The listing builds one solid part. Answer for the finished solid, in the listing's coordinates (mm). A direction names the side the tool comes from. Coordinates: 2 decimals unless noted, no trailing zeros. Order: outer loops, then holes, each group sorted by start corner. A loop starts at its lowest first (then second) coordinate and runs counter-clockwise, first axis right, second up. Notation, with made-up numbers: (65.25, -38) - (88.25, -38) arc R25 ccw to (88.25, -2) - close; hole circle Ø3 at (34.5, 67). An arc over 180 degrees is marked (long way). Use one line per item in the form item = value. Start each with the question number.
Item 1: Section B-B, the plane y = 9.75 is taken. Write down the section's boundary in (x, z).
Item 2: A tool of negligible diameter and unlimited length cuts with its end or side. For faces 1 (the flat face through (0, 10, -2)), 2 (the flat face through (0, -3, 0)), from which of +Z, -Z, +X, -X, +Y, -Y can it reach the whole face along a straight path? Write none if from no direction.
Item 3: Each of these flat-tipped pins is pushed along its axis until it touches: pin 1 Ø1.5 at (y, z) = (2, -1) entering from -X; pin 2 Ø3.5 at (x, y) = (0, 11) entering from -Z; pin 3 Ø1.1 at (x, z) = (1, -2.5) entering from +Y; pin 4 Ø3 at (y, z) = (7.5, 2) entering from +X. Where does it stop, or does it pass through?
Item 4: Consider line 1 along Y through (x, z) = (-1.5, -2.5); line 2 along Z through (x, y) = (2, 8.75); line 3 along X through (y, z) = (9, 2). Determine where each line is inside the solid, lowest interval first. Write a range as [from, to].
Item 5: Section A-A, the plane y = 2.25 is taken. Write down the section's boundary in (x, z).
Autodesk Inventor part; units mm, degrees
ref_plane "YZ Plane" through (0, 0, 0) normal (1, 0, 0) x (0, 1, 0)
ref_plane "XZ Plane" through (0, 0, 0) normal (0, 1, 0) x (-1, 0, 0)
ref_plane "XY Plane" through (0, 0, 0) normal (0, 0, 1) x (1, 0, 0)
sketch "スケッチ1" plane through (0, 0, 0) normal (0, 1, 0) x (-1, 0, 0)
  circle A0 centre (0, 0) radius 3
  dimension "d0" = 6
extrude "押し出し1" add sketch "スケッチ1" along normal blind 4
sketch "スケッチ2" plane through (0, 4, 0) normal (0, 1, 0) x (1, 0, 0)
  circle A0 centre (0, 0) radius 3
  line L0 (0, 3) -> (0, 2)
  line L1 (0, 2) -> (2.2361, 2)
  arc A1 (-2.2361, 2) -> (2.2361, 2) centre (0, 0) ccw
  line L2 (-2.2361, 2) -> (0, 2)
  dimension "d3" = 1
extrude "押し出し2" add sketch "スケッチ2" along normal blind 12 contours A0 L2 L1
sketch "スケッチ3" plane through (0, 0, 0) normal (0, -1, 0) x (1, 0, 0)
  circle A0 centre (0, 0) radius 3
extrude "押し出し3" add sketch "スケッチ3" along normal blind 3
fillet "フィレット1" radius 0.4 1 edges at (0, 16, 3)
properties part number "モーター100：1軸"
Response:
q1.outline = (-2.24, -2) - (2.24, -2) arc R3 ccw (long way) to start
q2.face_1 = -Z, +X, -X, +Y
q2.face_2 = +Z, -Z, +X, -X, -Y
q3.pin_1 = -2.99
q3.pin_2 = -2
q3.pin_3 = 16
q3.pin_4 = 2.96
q4.line_1 = [-3, 4]
q4.line_2 = [-2, 2.24]
q4.line_3 = [-2.24, 2.24]
q5.outline = circle Ø6 at (0, 0)
